Part model, mm, in its own coordinate system. A direction names the side the tool comes from. Round coordinates to 2 decimals unless told otherwise and drop trailing zeros. Write each loop counter-clockwise with the first axis right and the second up, starting at its lowest first coordinate (ties: lowest second). Pieces come first, ordered by that corner, then holes. Notation, with made-up numbers: M -14.75,74.25 L 24.25,74.25 A14 ccw 24.25,92.25 Z; hole C 84.25,20.5 d6. An arc over 180 degrees is marked long. Use a Markdown table: item, result. Add a question column.
1) Drop flat-ended pins along their axis: P1, Ø1, axis at x = 4.5, y = 18.5, coming from the +Z side; P2, Ø0.6, axis at x = 0.5, z = 4.5, coming from the -Y side; P3, Ø5, axis at x = -4.5, z = 1, coming from the +Y side; P4, Ø3, axis at y = 25.5, z = 2.5, coming from the +X side. Give the stop position or say it passes through.
2) Slice it at C-C on y = 14.25. Write the cut outline in (x, z), plus the area to 3 significant figures.
3) Slice it at A-A on x = 0. Write the cut outline in (y, z).
4) Slice it at B-B on z = -2.5. Write the cut outline in (x, y), plus the area to 3 significant figures.
5) Wall check: probe 1 along Y at (x, z) = (-4, -2); probe 2 along Z at (x, y) = (5, 7.25); probe 3 along Y at (x, z) = (2, -1.25). Give the ranges that are in metal, low to high.
6) Which spindle directions (+Z, -Z, +X, -X, +Y, -Y) get a long thin tool onto all of the face, cutting with end or side? Do faces 1 (the face through (5, 10, 0)), 2 (the face through (0, 5, 4)), 3 (the face through (-4.223, 11.232, 1.555)). Say none if no direction does.
```python
from build123d import *

# Parameters (mm, degrees)
ESQUISSE1_W        = 13
ESQUISSE1_H        = 8
BOSS_EXTRU_1_DEPTH = 10
ESQUISSE2_R        = 4.5
BOSS_EXTRU_2_DEPTH = 2.5
ESQUISSE3_R        = 2.9
BOSS_EXTRU_3_DEPTH = 8
ESQUISSE4_R        = 1.7
BOSS_EXTRU_4_DEPTH = 8
BOSS_EXTRU_4_TAPER = 4


with BuildPart() as part:
    # Esquisse1 → Boss.-Extru.1 (new body)
    with BuildSketch(Plane(origin=(0, 0, 0), x_dir=(1, 0, 0), z_dir=(0, 1, 0))):
        Rectangle(ESQUISSE1_W, ESQUISSE1_H)
    extrude(amount=BOSS_EXTRU_1_DEPTH)

    # Esquisse2 → Boss.-Extru.2 (add)
    with BuildSketch(Plane(origin=(0, 10, 0), x_dir=(1, 0, 0), z_dir=(0, 1, 0))):
        with Locations(Location((0, 0, 0), (0, 0, 62.733955549))):
            Circle(ESQUISSE2_R)
    extrude(amount=BOSS_EXTRU_2_DEPTH)

    # Esquisse3 → Boss.-Extru.3 (add)
    with BuildSketch(Plane(origin=(0, 12.5, 0), x_dir=(1, 0, 0), z_dir=(0, 1, 0))):
        with Locations(Location((0, 0, 0), (0, 0, 270))):
            Circle(ESQUISSE3_R)
    extrude(amount=BOSS_EXTRU_3_DEPTH)

    # Esquisse4 → Boss.-Extru.4 (add)
    with BuildSketch(Plane(origin=(0, 20.5, 0), x_dir=(1, 0, 0), z_dir=(0, 1, 0))):
        Circle(ESQUISSE4_R)
    extrude(amount=BOSS_EXTRU_4_DEPTH, taper=BOSS_EXTRU_4_TAPER)


solid = part.part
```
Entries:
| question | item | result |
|---|---|---|
| 1 | P1 | passes through |
| 1 | P2 | stops at y = 10 |
| 1 | P3 | stops at y = 20.5 |
| 1 | P4 | stops at x = 0.91 |
| 2 | outline | C 0,0 d5.8 |
| 2 | area | 26.4 mm^2 |
| 3 | outline | M 0,-4 L 10,-4 L 10,-4.5 L 12.5,-4.5 L 12.5,-2.9 L 20.5,-2.9 L 20.5,-1.7 L 28.5,-1.14 L 28.5,1.14 L 20.5,1.7 L 20.5,2.9 L 12.5,2.9 L 12.5,4.5 L 10,4.5 L 10,4 L 0,4 Z |
| 4 | outline | M -6.5,0 L 6.5,0 L 6.5,10 L 3.74,10 L 3.74,12.5 L 1.47,12.5 L 1.47,20.5 L -1.47,20.5 L -1.47,12.5 L -3.74,12.5 L -3.74,10 L -6.5,10 Z |
| 4 | area | 172 mm^2 |
| 5 | probe 1 | y = 0 to 12.5 |
| 5 | probe 2 | z = -4 to 4 |
| 5 | probe 3 | y = 0 to 20.5 |
| 6 | face 1 | +X, +Y |
| 6 | face 2 | +Z, +X, -X, -Y |
| 6 | face 3 | +Y |
